```python
from build123d import *

# Parameters (mm, degrees)
ESQUISSE1_W             = 20
ESQUISSE1_H             = 10
BOSS_EXTRU_1_DEPTH      = 20
ESQUISSE2_R             = 1.75
ENL_V_MAT_EXTRU_1_DEPTH = 31
ESQUISSE3_R             = 1.75
ENL_V_MAT_EXTRU_2_DEPTH = 40
ESQUISSE4_R             = 1.75
ENL_V_MAT_EXTRU_3_DEPTH = 40


with BuildPart() as part:
    # Esquisse1 → Boss.-Extru.1 (new body)
    with BuildSketch(Plane(origin=(0, 0, 0), x_dir=(0, 0, -1), z_dir=(1, 0, 0))):
        with Locations((10, 5)):
            Rectangle(ESQUISSE1_W, ESQUISSE1_H)
    extrude(amount=BOSS_EXTRU_1_DEPTH)

    # Esquisse2 → Enlèv. mat.-Extru.1 (cut, through all)
    with BuildSketch(Plane(origin=(0, 10, 0), x_dir=(1, 0, 0), z_dir=(0, 1, 0))):
        with Locations(Location((5, 15, 0), (0, 0, 270))):
            Circle(ESQUISSE2_R)
        with Locations(Location((15, 15, 0), (0, 0, 270))):
            Circle(ESQUISSE2_R)
        with Locations((25, 15)):
            Circle(ESQUISSE2_R)
        with Locations((35, 15)):
            Circle(ESQUISSE2_R)
        with Locations(Location((5, 5, 0), (0, 0, 270))):
            Circle(ESQUISSE2_R)
        with Locations(Location((15, 5, 0), (0, 0, 270))):
            Circle(ESQUISSE2_R)
        with Locations((25, 5)):
            Circle(ESQUISSE2_R)
        with Locations((35, 5)):
            Circle(ESQUISSE2_R)
        with Locations((5, -5)):
            Circle(ESQUISSE2_R)
        with Locations((15, -5)):
            Circle(ESQUISSE2_R)
        with Locations((25, -5)):
            Circle(ESQUISSE2_R)
        with Locations((35, -5)):
            Circle(ESQUISSE2_R)
        with Locations((5, -15)):
            Circle(ESQUISSE2_R)
        with Locations((15, -15)):
            Circle(ESQUISSE2_R)
        with Locations((25, -15)):
            Circle(ESQUISSE2_R)
        with Locations((35, -15)):
            Circle(ESQUISSE2_R)
    extrude(amount=-ENL_V_MAT_EXTRU_1_DEPTH, mode=Mode.SUBTRACT)

    # Esquisse3 → Enlèv. mat.-Extru.2 (cut)
    with BuildSketch(Plane.XY):
        with Locations((5, 5)):
            Circle(ESQUISSE3_R)
        with Locations((15, 5)):
            Circle(ESQUISSE3_R)
        with Locations((25, 5)):
            Circle(ESQUISSE3_R)
        with Locations((35, 5)):
            Circle(ESQUISSE3_R)
    extrude(amount=-ENL_V_MAT_EXTRU_2_DEPTH, mode=Mode.SUBTRACT)

    # Esquisse4 → Enlèv. mat.-Extru.3 (cut)
    with BuildSketch(Plane(origin=(20, 0, 0), x_dir=(0, 0, -1), z_dir=(1, 0, 0))):
        with Locations((5, 5)):
            Circle(ESQUISSE4_R)
        with Locations(Location((15, 5, 0), (0, 0, 315))):
            Circle(ESQUISSE4_R)
        with Locations((25, 5)):
            Circle(ESQUISSE4_R)
        with Locations((35, 5)):
            Circle(ESQUISSE4_R)
    extrude(amount=-ENL_V_MAT_EXTRU_3_DEPTH, mode=Mode.SUBTRACT)


solid = part.part
```
The model under review builds one solid part; all positions refer to its coordinate system, in mm. Round coordinates to 2 decimals unless told otherwise and drop trailing zeros. Loops run counter-clockwise (first coordinate to the right, second up) from the corner with the lowest first, then second, coordinate; pieces in that order, holes last. Notation, with made-up numbers: M 59.5,2.5 L 103.5,2.5 A24 cw 103.5,23.5 Z; hole C -17.75,19.25 d9. An arc over 180 degrees is marked long. Write item = value, one per line.
Item 1: For line 1 (X direction, y = 5, z = -8.5); line 2 (Z direction, x = 5, y = 2.6); line 3 (Z direction, x = 10.25, y = 4.25), list the stretches that pass through material, from the lowest coordinate up. Write a range as [from, to].
Return value:
line_1 = [0, 3.25], [6.75, 13.25], [16.75, 20]
line_2 = [-20, -16.75], [-13.25, -6.75], [-3.25, 0]
line_3 = [-20, -16.58], [-13.42, -6.58], [-3.42, 0]
Item 2: Take a section at C-C on y = 8.5. Write out the cut boundary in (x, z).
Return value:
outline = M 0,-20 L 20,-20 L 20,0 L 0,0 Z; hole C 5,-15 d3.5; hole C 5,-5 d3.5; hole C 15,-15 d3.5; hole C 15,-5 d3.5
Item 3: Take a section at D-D on z = -10. Write out the cut boundary in (x, y), then the cut area to 3 significant figures.
Return value:
outline = M 0,0 L 20,0 L 20,10 L 0,10 Z; hole C 5,5 d3.5; hole C 15,5 d3.5
area = 181 mm2
Item 4: Take a section at B-B on x = 15. Write out the cut boundary in (y, z).
Return value:
outline = M 0,-20 L 3.25,-20 L 3.25,-16.75 L 0,-16.75 Z; M 0,-13.25 L 3.25,-13.25 L 3.25,-6.75 L 0,-6.75 Z; M 0,-3.25 L 3.25,-3.25 L 3.25,0 L 0,0 Z; M 6.75,-20 L 10,-20 L 10,-16.75 L 6.75,-16.75 Z; M 6.75,-13.25 L 10,-13.25 L 10,-6.75 L 6.75,-6.75 Z; M 6.75,-3.25 L 10,-3.25 L 10,0 L 6.75,0 Z
Item 5: Insertion check: P1, Ø4, axis at y = 5, z = -15, coming from the +X side; P2, Ø3, axis at x = 15, y = 5, coming from the +Z side. Each pin has a flat end and moves straight along its axis. Give the tip position at first contact, or say it passes through.
Return value:
P1 = 20
P2 = through
Item 6: Take a section at A-A on z = -15. Write out the cut boundary in (x, y), then the cut area to 3 significant figures.
Return value:
outline = M 0,0 L 3.25,0 L 3.25,3.25 L 0,3.25 Z; M 0,6.75 L 3.25,6.75 L 3.25,10 L 0,10 Z; M 6.75,0 L 13.25,0 L 13.25,3.25 L 6.75,3.25 Z; M 6.75,6.75 L 13.25,6.75 L 13.25,10 L 6.75,10 Z; M 16.75,0 L 20,0 L 20,3.25 L 16.75,3.25 Z; M 16.75,6.75 L 20,6.75 L 20,10 L 16.75,10 Z
area = 84.5 mm2
Item 7: The part is to be moulded in two halves that separate along Z. For faces 1 (the flat face through (10, 5, -20)), 2 (the cylindrical face through (13.25, 5.08, -1.85)), 3 (the cylindrical face through (15.08, 8.15, -6.75)), say which applies: released by +Z, released by -Z, zero draft, split by the parting line, or undercut.
Return value:
face_1 = released by -Z
face_2 = zero draft
face_3 = undercut
